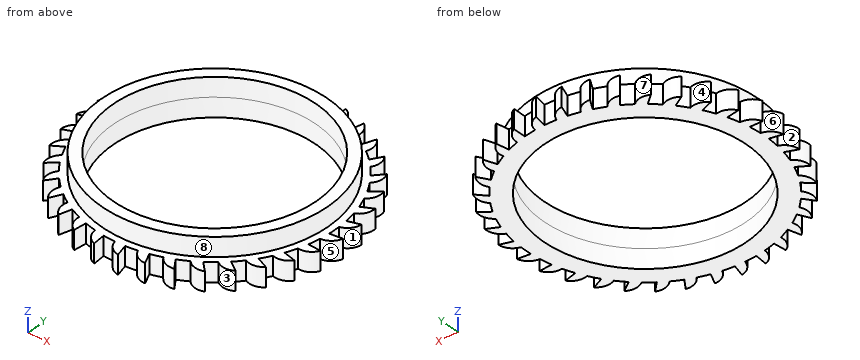
```python
from build123d import *

# Parameters (mm, degrees)
BOSS_EXTRUDE1_DEPTH = 10
SKETCH2_R           = 59.5
SKETCH2_R_2         = 53.5
BOSS_EXTRUDE2_DEPTH = 10
SKETCH3_R           = 53.5
CUT_EXTRUDE4_DEPTH  = 10


with BuildPart() as part:
    # Sketch1 → Boss-Extrude1 (new body)
    with BuildSketch(Plane.XY):
        with BuildLine():
            Line((0, 69.588014501), (1.048611539, 62.991272521))
            ThreePointArc((1.048611539, 62.991272521), (-2.021331039, 62.967564832), (-5.0864736, 62.794329253))
            ThreePointArc((-5.0864736, 62.794329253), (-7.836974129, 66.820360054), (-12.425419784, 68.469706479))
            Line((-12.425419784, 68.469706479), (-10.2157661, 62.166213677))
            ThreePointArc((-10.2157661, 62.166213677), (-13.232140267, 61.594727566), (-16.217092319, 60.876973617))
            ThreePointArc((-16.217092319, 60.876973617), (-19.642266731, 64.347183613), (-24.451476353, 65.150725754))
            Line((-24.451476353, 65.150725754), (-21.151800612, 59.343081576))
            ThreePointArc((-21.151800612, 59.343081576), (-24.017657619, 58.242185077), (-26.826480348, 57.002981958))
            ThreePointArc((-26.826480348, 57.002981958), (-30.816240719, 59.805835745), (-35.691642354, 59.737747098))
            Line((-35.691642354, 59.737747098), (-31.407998848, 54.612614004))
            ThreePointArc((-31.407998848, 54.612614004), (-34.031227694, 53.017690837), (-36.573643225, 51.296867558))
            ThreePointArc((-36.573643225, 51.296867558), (-40.999755374, 53.342279108), (-45.784649601, 52.404748097))
            Line((-45.784649601, 52.404748097), (-40.654718159, 48.126852083))
            ThreePointArc((-40.654718159, 48.126852083), (-42.951006109, 46.08916439), (-45.145299116, 43.942029627))
            ThreePointArc((-45.145299116, 43.942029627), (-49.865504157, 45.164257731), (-54.406100539, 43.387417373))
            Line((-54.406100539, 43.387417373), (-48.594761377, 40.094253538))
            ThreePointArc((-48.594761377, 40.094253538), (-50.490303849, 37.679294278), (-52.265947947, 35.174858708))
            ThreePointArc((-52.265947947, 35.174858708), (-57.128534607, 35.534619949), (-61.27889464, 32.975579356))
            Line((-61.27889464, 32.975579356), (-54.97292898, 30.772992693))
            ThreePointArc((-54.97292898, 30.772992693), (-56.406801678, 28.058380645), (-57.706726208, 25.277138889))
            ThreePointArc((-57.706726208, 25.277138889), (-62.555406949, 24.762870243), (-66.182134647, 21.503879086))
            Line((-66.182134647, 21.503879086), (-59.584221415, 20.462662544))
            ThreePointArc((-59.584221415, 20.462662544), (-60.510338491, 17.535647571), (-61.292762806, 14.566991027))
            ThreePointArc((-61.292762806, 14.566991027), (-65.97169704, 13.195221514), (-68.958226392, 9.341026448))
            Line((-68.958226392, 9.341026448), (-62.280427947, 9.494645584))
            ThreePointArc((-62.280427947, 9.494645584), (-62.669023236, 6.449304357), (-62.908799576, 3.388648088))
            ThreePointArc((-62.908799576, 3.388648088), (-67.267602508, 1.203467507), (-69.517944001, -3.122054465))
            Line((-69.517944001, -3.122054465), (-62.97489028, -1.778537098))
            ThreePointArc((-62.97489028, -1.778537098), (-62.81347401, -4.844324807), (-62.502895767, -7.898608789))
            ThreePointArc((-62.502895767, -7.898608789), (-66.401471883, -10.826966935), (-67.84329769, -15.484789979))
            Line((-67.84329769, -15.484789979), (-61.645287824, -12.994556134))
            ThreePointArc((-61.645287824, -12.994556134), (-60.939048046, -15.982253385), (-60.088097459, -18.93199788))
            ThreePointArc((-60.088097459, -18.93199788), (-63.401143316, -22.509413752), (-63.98811197, -27.349831602))
            Line((-63.98811197, -27.349831602), (-58.334355095, -23.792919443))
            ThreePointArc((-58.334355095, -23.792919443), (-57.105990937, -26.606499189), (-55.742018259, -29.356896982))
            ThreePointArc((-55.742018259, -29.356896982), (-58.363049836, -33.468389489), (-58.076295682, -38.335827134))
            Line((-58.076295682, -38.335827134), (-53.148508196, -33.826558745))
            ThreePointArc((-53.148508196, -33.826558745), (-51.437500293, -36.375590217), (-49.604344727, -38.83824126))
            ThreePointArc((-49.604344727, -38.83824126), (-51.449119914, -43.351663651), (-50.297859465, -48.089677639))
            Line((-50.297859465, -48.089677639), (-46.254424513, -42.772984617))
            ThreePointArc((-46.254424513, -42.772984617), (-44.115766066, -44.975539846), (-41.872346741, -47.071292508))
            ThreePointArc((-41.872346741, -47.071292508), (-42.881572944, -51.841579673), (-40.90280866, -56.297886336))
            Line((-40.90280866, -56.297886336), (-37.873685567, -50.344651569))
            ThreePointArc((-37.873685567, -50.344651569), (-35.376114819, -52.129938618), (-32.794537078, -53.791433684))
            ThreePointArc((-32.794537078, -53.791433684), (-32.935776938, -58.665264669), (-30.193107929, -62.696634645))
            Line((-30.193107929, -62.696634645), (-28.275655205, -56.298199996))
            ThreePointArc((-28.275655205, -56.298199996), (-25.499446135, -57.60883827), (-22.66268401, -58.782673922))
            ThreePointArc((-22.66268401, -58.782673922), (-21.931397961, -63.603399789), (-18.512975867, -67.080261528))
            Line((-18.512975867, -67.080261528), (-17.768822019, -60.442277952))
            ThreePointArc((-17.768822019, -60.442277952), (-14.80320427, -61.23614246), (-11.802433631, -61.884590654))
            ThreePointArc((-11.802433631, -61.884590654), (-10.222125808, -66.497269306), (-6.237821528, -69.307873613))
            Line((-6.237821528, -69.307873613), (-6.690884273, -62.643691363))
            ThreePointArc((-6.690884273, -62.643691363), (-3.631175241, -62.895266645), (-0.562843324, -62.997485723))
            ThreePointArc((-0.562843324, -62.997485723), (1.815693879, -67.253861874), (6.237821528, -69.307873613))
            Line((6.237821528, -69.307873613), (4.602103998, -62.831684991))
            ThreePointArc((4.602103998, -62.831684991), (7.657562749, -62.53288521), (10.69483723, -62.085589766))
            ThreePointArc((10.69483723, -62.085589766), (13.795155671, -65.848859984), (18.512975867, -67.080261528))
            Line((18.512975867, -67.080261528), (15.74717686, -61.000216565))
            ThreePointArc((15.74717686, -61.000216565), (18.700180371, -60.160645393), (21.608776916, -59.17821187))
            ThreePointArc((21.608776916, -59.17821187), (25.331229809, -62.327421554), (30.193107929, -62.696634645))
            Line((30.193107929, -62.696634645), (26.386122502, -57.208150987))
            ThreePointArc((26.386122502, -57.208150987), (29.14175881, -55.854792932), (31.828192733, -54.368797553))
            ThreePointArc((31.828192733, -54.368797553), (36.053137378, -56.802728512), (40.90280866, -56.297886336))
            Line((40.90280866, -56.297886336), (36.176996455, -51.577368365))
            ThreePointArc((36.176996455, -51.577368365), (38.646697142, -49.753721469), (41.024624246, -47.811925348))
            ThreePointArc((41.024624246, -47.811925348), (45.616267447, -49.452349038), (50.297859465, -48.089677639))
            Line((50.297859465, -48.089677639), (44.805111976, -44.288846686))
            ThreePointArc((44.805111976, -44.288846686), (46.90949883, -42.05352446), (48.902490582, -39.718338522))
            ThreePointArc((48.902490582, -39.718338522), (53.713253147, -40.512530377), (58.076295682, -38.335827134))
            Line((58.076295682, -38.335827134), (51.993154332, -35.576845034))
            ThreePointArc((51.993154332, -35.576845034), (53.664590628, -33.001692573), (55.208590632, -30.348171615))
            ThreePointArc((55.208590632, -30.348171615), (60.083850696, -30.270605655), (63.98811197, -27.349831602))
            Line((63.98811197, -27.349831602), (57.510093928, -25.72137431))
            ThreePointArc((57.510093928, -25.72137431), (58.694858328, -22.889159134), (59.740241154, -20.002589503))
            ThreePointArc((59.740241154, -20.002589503), (64.523303846, -19.055758761), (67.84329769, -15.484789979))
            Line((67.84329769, -15.484789979), (61.178611786, -15.039197451))
            ThreePointArc((61.178611786, -15.039197451), (61.838624987, -12.040949286), (62.351791171, -9.014107705))
            ThreePointArc((62.351791171, -9.014107705), (66.888924921, -7.228444101), (69.517944001, -3.122054465))
            Line((69.517944001, -3.122054465), (62.880798722, -3.873648413))
            ThreePointArc((62.880798722, -3.873648413), (62.994847358, -0.805733421), (62.959303317, 2.264094931))
            ThreePointArc((62.959303317, 2.264094931), (67.104680912, 4.8311987), (68.958226392, 9.341026448))
            Line((68.958226392, 9.341026448), (62.56194505, 7.416402873))
            ThreePointArc((62.56194505, 7.416402873), (62.126363502, 10.455379379), (61.543251651, 13.469527693))
            ThreePointArc((61.543251651, 13.469527693), (65.163637245, 16.735562799), (66.182134647, 21.503879086))
            Line((66.182134647, 21.503879086), (60.232298987, 18.468084869))
            ThreePointArc((60.232298987, 18.468084869), (59.261087206, 21.380447683), (58.149149238, 24.242038752))
            ThreePointArc((58.149149238, 24.242038752), (61.12818066, 28.10203214), (61.27889464, 32.975579356))
            Line((61.27889464, 32.975579356), (55.966737276, 28.926187421))
            ThreePointArc((55.966737276, 28.926187421), (54.491110807, 31.618330807), (52.886085324, 34.235390739))
            ThreePointArc((52.886085324, 34.235390739), (55.128014052, 38.565279046), (54.406100539, 43.387417373))
            Line((54.406100539, 43.387417373), (49.902358579, 38.454578509))
            ThreePointArc((49.902358579, 38.454578509), (47.969745271, 40.839974763), (45.923219113, 43.128389099))
            ThreePointArc((45.923219113, 43.128389099), (47.355987713, 47.789006151), (45.784649601, 52.404748097))
            Line((45.784649601, 52.404748097), (42.234077017, 46.747007803))
            ThreePointArc((42.234077017, 46.747007803), (39.906592652, 48.748988327), (37.484342854, 50.635205547))
            ThreePointArc((37.484342854, 50.635205547), (38.061900964, 55.476755278), (35.691642354, 59.737747098))
            Line((35.691642354, 59.737747098), (33.20835747, 53.536949802))
            ThreePointArc((33.20835747, 53.536949802), (30.560809311, 55.091169295), (27.840688973, 56.514564826))
            ThreePointArc((27.840688973, 56.514564826), (27.544473401, 61.381435844), (24.451476353, 65.150725754))
            Line((24.451476353, 65.150725754), (23.11529399, 58.606170185))
            ThreePointArc((23.11529399, 58.606170185), (20.232776412, 59.662674753), (17.302212441, 60.577499491))
            ThreePointArc((17.302212441, 60.577499491), (16.141743799, 65.313266557), (12.425419784, 68.469706479))
            Line((12.425419784, 68.469706479), (12.279285941, 61.791740037))
            ThreePointArc((12.279285941, 61.791740037), (9.254445432, 62.316572754), (6.207628565, 62.69342348))
            ThreePointArc((6.207628565, 62.69342348), (4.22020527, 67.145875143), (0, 69.588014501))
        make_face()
    extrude(amount=BOSS_EXTRUDE1_DEPTH)

    # Sketch2 → Boss-Extrude2 (add)
    with BuildSketch(Plane.XY.offset(10)):
        with Locations(Location((0, 0, 0), (0, 0, 180))):  # turned: the seam where the file's is
            Circle(SKETCH2_R)
        Circle(SKETCH2_R_2, mode=Mode.SUBTRACT)
    extrude(amount=BOSS_EXTRUDE2_DEPTH)

    # Sketch3 → Cut-Extrude4 (cut)
    with BuildSketch(Plane.XY.offset(10)):
        Circle(SKETCH3_R)
    extrude(amount=-CUT_EXTRUDE4_DEPTH, mode=Mode.SUBTRACT)


solid = part.part
```
Input: part model. Units: mm. Frame: model coordinates. Face numbers are marked on the shaded views. A direction names the side the tool comes from. Coordinates: 2 decimals unless noted, no trailing zeros. Write each loop counter-clockwise with the first axis right and the second up, starting at its lowest first coordinate (ties: lowest second). Pieces come first, ordered by that corner, then holes. Notation, with made-up numbers: (-29, -13) - (-8, -13) arc R15 ccw to (-8, 4) - close; hole circle Ø8 at (74, 1.25). An arc over 180 degrees is marked (long way). Put each result on its own line as item: value. Start each with the question number.
1) Reachability of the marked faces 4, 5, 6, 7 and 8 from +Z, -Z, +X, -X, +Y, -Y: full face, straight path, thin tool, end or side. Return the list, or none.
2) Ray query, L1, parallel to Y at x = 0, z = 16; L2, parallel to Y at x = 36.5, z = 18.75; L3, parallel to X at y = -46.5, z = 19. Return the intervals inside material, ascending.
3) Mould query, pull axis X, two halves, no side actions, for the marked faces 1, 2 and 3. Classes: pulls with the +X half, pulls with the -X half, needs draft (parallel to the pull), parting line crosses it, or undercut.
4) Cut plane A-A (y = 0). Return the cut outline in (x, z).
5) Cut plane B-B (z = 15.5). Return the cut outline in (x, y).
6) Contact query for flat-ended pins moving along their axis: pin 1 (8 mm diameter, centred on x = 28.5, z = 13, fed in from -Y); pin 2 (10 mm diameter, centred on y = -48, z = 5.5, fed in from -X); pin 3 (1 mm diameter, centred on x = -46, z = 12, fed in from -Y). Output: stop coordinate, or through.
Resolved:
1. face 4: +Z, -Z
1. face 5: +Z, -Z, +X
1. face 6: +Z, -Z, -X
1. face 7: +Z, -Z, +Y
1. face 8: +Z
2. L1: y = -59.5 to -53.5, 53.5 to 59.5
2. L2: y = -46.99 to -39.12, 39.12 to 46.99
2. L3: x = -37.12 to -26.46, 26.46 to 37.12
3. face 1: pulls with the +X half
3. face 2: pulls with the -X half
3. face 3: undercut
4. outline: (-68.27, 0) - (-53.5, 0) - (-53.5, 20) - (-59.5, 20) - (-59.5, 10) - (-68.27, 10) - close; (53.5, 0) - (63, 0) - (63, 10) - (59.5, 10) - (59.5, 20) - (53.5, 20) - close
5. outline: circle Ø119 at (0, 0); hole circle Ø107 at (0, 0)
6. pin 1: stops at y = -62.92
6. pin 2: stops at x = -51.47
6. pin 3: stops at y = -38.34
